CAD build for the part. Positions are in the model's coordinates, mm. Give positions to 0.01 mm unless a question says otherwise; leave off trailing zeros. Order: outer loops, then holes, each group sorted by start corner. A loop starts at its lowest first (then second) coordinate and runs counter-clockwise, first axis right, second up.
Item 1: Band-saw the part on B-B on x = 101. Give the cut face in (y, z).
Item 2: Wall check: L1, parallel to Z at x = -4, y = -122; L2, parallel to Y at x = 6.5, z = -26.5; L3, parallel to Z at x = 77, y = -20. Give the ranges that are in metal, low to high.
Item 3: Band-saw the part on A-A on z = 31. Give the cut face in (x, y).
Item 4: Flat gauge pins, fed straight in: P1, Ø4, axis at x = -66.5, z = 5.5, coming from the -Y side; P2, Ø2, axis at x = -28, z = -63, coming from the -Y side; P3, Ø10, axis at x = -95, y = 31, coming from the -Z side. Where does each tip first touch, or does it go through?
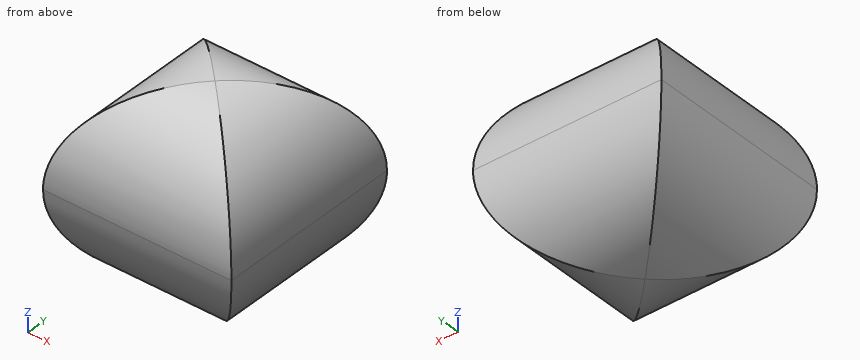
```python
from build123d import *
from build123d import SkipClean  # not in build123d's __all__

# Parameters (mm, degrees)
F0_W     = 304.8
F0_H     = 304.8
F1_DEPTH = 152.4
F2_R     = 152.4
F4_DEPTH = 152.4
F3_R     = 152.4
F5_DEPTH = 152.4


with BuildPart() as f1:
    # F0 (on Top) → F1 (new body, symmetric)
    with BuildSketch(Plane.XY):
        Rectangle(F0_W, F0_H)
    extrude(amount=F1_DEPTH, both=True)

    # F2 (on Right) → F4 (intersect, symmetric)
    with BuildSketch(Plane.YZ):
        Circle(F2_R)
    extrude(amount=F4_DEPTH, both=True, mode=Mode.INTERSECT)

    # F3 (on Front) → F5 (intersect, symmetric)
    with BuildSketch(Plane.XZ):
        Circle(F3_R)
    with SkipClean():  # cleaning this boolean's faces spoils the solid; the shape is the same uncleaned
        extrude(amount=F5_DEPTH, both=True, mode=Mode.INTERSECT)


solid = f1.part
```
The answers:
1. outline: (-101, -114.13) - (101, -114.13) arc R152.4 ccw to (101, 114.13) - (-101, 114.13) arc R152.4 ccw to start
2. L1: z = -91.33 to 91.33
2. L2: y = -150.08 to 150.08
2. L3: z = -131.52 to 131.52
3. outline: (-149.21, -149.21) - (149.21, -149.21) - (149.21, 149.21) - (-149.21, 149.21) - close
4. P1: stops at y = -152.36
4. P2: stops at y = -139.22
4. P3: stops at z = -122.99
